Can you work these out from the model? Positions are in its coordinate system, mm. A direction names the side the tool comes from. Round coordinates to 2 decimals unless told otherwise and drop trailing zeros. Loops run counter-clockwise (first coordinate to the right, second up) from the corner with the lowest first, then second, coordinate; pieces in that order, holes last. Notation, with made-up numbers: M 56.25,62.5 L 104.25,62.5 A22 cw 104.25,87.5 Z; hole C 33.5,55.25 d1. An arc over 180 degrees is marked long. Return JSON: item names as keys, results as strings.
```python
from build123d import *

# Parameters (mm, degrees)
SKETCH_1_W             = 760
SKETCH_1_H             = 160
EXTRUDE_1_DEPTH        = 10
SKETCH_2_R             = 19
CUT_EXTRUDE_1_DEPTH    = 777.916983982
CUT_EXTRUDE_2_DEPTH    = 2
CUT_EXTRUDE_4_DEPTH    = 2.7
CUT_EXTRUDE_5_DEPTH    = 777.868071168
HOLE_WIZARD_M6_1_D     = 5
HOLE_WIZARD_M6_1_DEPTH = 15
HOLE_WIZARD_M6_1_TIP   = 1.502151548
FILLET_1_R             = 0.13
FILLET_2_R             = 0.5
FILLET_3_R             = 0.5
FILLET_4_R             = 0.13


with BuildPart() as part:
    # 스케치1 → 보스-돌출1 (new, symmetric)
    with BuildSketch(Plane(origin=(0, 0, 0), x_dir=(1, 0, 0), z_dir=(0, 1, 0))):
        with Locations((380, 80)):
            Rectangle(SKETCH_1_W, SKETCH_1_H)
    extrude(amount=EXTRUDE_1_DEPTH, both=True)

    # 스케치2 → 컷-돌출1 (cut, through all)
    with BuildSketch(Plane(origin=(0, 10, 0), x_dir=(1, 0, 0), z_dir=(0, 1, 0))):
        with Locations(Location((280, 80, 0), (0, 0, 270))):
            Circle(SKETCH_2_R)
        with Locations(Location((380, 80, 0), (0, 0, 270))):
            Circle(SKETCH_2_R)
    extrude(amount=-CUT_EXTRUDE_1_DEPTH, mode=Mode.SUBTRACT)

    # 스케치3 → 컷-돌출2 (cut)
    with BuildSketch(Plane(origin=(0, 10, 0), x_dir=(1, 0, 0), z_dir=(0, 1, 0))):
        with BuildLine():
            Line((520.5, 146), (679.5, 146))
            ThreePointArc((679.5, 146), (694.349242405, 139.849242405), (700.5, 125))
            Line((700.5, 125), (700.5, 66))
            ThreePointArc((700.5, 66), (694.349242405, 51.150757595), (679.5, 45))
            Line((679.5, 45), (520.5, 45))
            ThreePointArc((520.5, 45), (505.650757595, 51.150757595), (499.5, 66))
            Line((499.5, 66), (499.5, 125))
            ThreePointArc((499.5, 125), (505.650757595, 139.849242405), (520.5, 146))
        make_face()
    extrude(amount=-CUT_EXTRUDE_2_DEPTH, mode=Mode.SUBTRACT)

    # 스케치4 → 컷-돌출4 (cut)
    with BuildSketch(Plane(origin=(0, 8, 0), x_dir=(1, 0, 0), z_dir=(0, 1, 0))):
        with BuildLine():
            Line((532.5, 124.55), (667.5, 124.55))
            ThreePointArc((667.5, 124.55), (676.020636713, 121.020636713), (679.55, 112.5))
            Line((679.55, 112.5), (679.55, 77.5))
            ThreePointArc((679.55, 77.5), (676.020636713, 68.979363287), (667.5, 65.45))
            Line((667.5, 65.45), (532.5, 65.45))
            ThreePointArc((532.5, 65.45), (523.979363287, 68.979363287), (520.45, 77.5))
            Line((520.45, 77.5), (520.45, 112.5))
            ThreePointArc((520.45, 112.5), (523.979363287, 121.020636713), (532.5, 124.55))
        make_face()
        with BuildLine():
            Line((532.5, 120.45), (667.5, 120.45))
            ThreePointArc((667.5, 120.45), (673.12149891, 118.12149891), (675.45, 112.5))
            Line((675.45, 112.5), (675.45, 77.5))
            ThreePointArc((675.45, 77.5), (673.12149891, 71.87850109), (667.5, 69.55))
            Line((667.5, 69.55), (532.5, 69.55))
            ThreePointArc((532.5, 69.55), (526.87850109, 71.87850109), (524.55, 77.5))
            Line((524.55, 77.5), (524.55, 112.5))
            ThreePointArc((524.55, 112.5), (526.87850109, 118.12149891), (532.5, 120.45))
        make_face(mode=Mode.SUBTRACT)
    extrude(amount=-CUT_EXTRUDE_4_DEPTH, mode=Mode.SUBTRACT)

    # 스케치5 → 컷-돌출5 (cut, through all)
    with BuildSketch(Plane(origin=(0, 8, 0), x_dir=(1, 0, 0), z_dir=(0, 1, 0))):
        with BuildLine():
            Line((534.5, 116), (665.5, 116))
            ThreePointArc((665.5, 116), (669.035533906, 114.535533906), (670.5, 111))
            Line((670.5, 111), (670.5, 80))
            ThreePointArc((670.5, 80), (669.035533906, 76.464466094), (665.5, 75))
            Line((665.5, 75), (534.5, 75))
            ThreePointArc((534.5, 75), (530.964466094, 76.464466094), (529.5, 80))
            Line((529.5, 80), (529.5, 111))
            ThreePointArc((529.5, 111), (530.964466094, 114.535533906), (534.5, 116))
        make_face()
    extrude(amount=-CUT_EXTRUDE_5_DEPTH, mode=Mode.SUBTRACT)

    # M6 나사 구멍1
    with Locations(Plane(origin=(0, 8, 0), x_dir=(1, 0, 0), z_dir=(0, 1, 0))):
        with Locations((530, 135.5), (600, 135.5), (670, 135.5), (670, 54.5), (600, 54.5), (530, 54.5), (509.5, 95), (690.5, 95)):
            Hole(HOLE_WIZARD_M6_1_D / 2, depth=HOLE_WIZARD_M6_1_DEPTH)
            with Locations((0, 0, -(HOLE_WIZARD_M6_1_DEPTH + HOLE_WIZARD_M6_1_TIP / 2))):  # 118° drill point
                Cone(0, HOLE_WIZARD_M6_1_D / 2, HOLE_WIZARD_M6_1_TIP, mode=Mode.SUBTRACT)

    # 필렛1
    fillet_1_edges = [part.edges().sort_by_distance(p)[0] for p in [
        (523.979363287, 8, -121.020636713),
        (520.45, 8, -95),
        (523.979363287, 8, -68.979363287),
        (600, 8, -65.45),
        (676.020636713, 8, -68.979363287),
        (679.55, 8, -95),
        (676.020636713, 8, -121.020636713),
        (600, 8, -124.55),
    ]]
    fillet(fillet_1_edges, radius=FILLET_1_R)

    # 필렛2
    fillet_2_edges = [part.edges().sort_by_distance(p)[0] for p in [
        (523.979363287, 5.3, -121.020636713),
        (600, 5.3, -124.55),
        (676.020636713, 5.3, -121.020636713),
        (679.55, 5.3, -95),
        (676.020636713, 5.3, -68.979363287),
        (600, 5.3, -65.45),
        (523.979363287, 5.3, -68.979363287),
        (520.45, 5.3, -95),
    ]]
    fillet(fillet_2_edges, radius=FILLET_2_R)

    # 필렛3
    fillet_3_edges = [part.edges().sort_by_distance(p)[0] for p in [
        (675.45, 5.3, -95),
        (673.12149891, 5.3, -118.12149891),
        (600, 5.3, -120.45),
        (526.87850109, 5.3, -118.12149891),
        (524.55, 5.3, -95),
        (526.87850109, 5.3, -71.87850109),
        (600, 5.3, -69.55),
        (673.12149891, 5.3, -71.87850109),
    ]]
    fillet(fillet_3_edges, radius=FILLET_3_R)

    # 필렛4
    fillet_4_edges = [part.edges().sort_by_distance(p)[0] for p in [
        (673.12149891, 8, -118.12149891),
        (675.45, 8, -95),
        (673.12149891, 8, -71.87850109),
        (600, 8, -69.55),
        (526.87850109, 8, -71.87850109),
        (524.55, 8, -95),
        (526.87850109, 8, -118.12149891),
        (600, 8, -120.45),
    ]]
    fillet(fillet_4_edges, radius=FILLET_4_R)


solid = part.part
```
Q1. Suppose I cut it at C-C, the plane x = 368.5. Please give me the cut outline in (y, z).
Results:
{"outline": "M -10,-160 L 10,-160 L 10,-95.12 L -10,-95.12 Z; M -10,-64.88 L 10,-64.88 L 10,0 L -10,0 Z"}
Q2. Thinking about a two-plate mould opening in X: for faces 4 (the cylindrical face through (524.07, 6.85, -68.89)), 5 (the cylindrical face through (505.488, 9.014, -139.685)), 6 (the flat face through (0, 0, -79)), 7 (the flat face through (375, 0, -160)), which applies, pulls with the +X half, pulls with the -X half, needs draft (parallel to the pull), parting line crosses it, or undercut?
Results:
{"face 4": "undercut", "face 5": "undercut", "face 6": "pulls with the -X half", "face 7": "needs draft"}
Q3. Suppose I cut it at A-A, the plane y = -3.75. State how many separate pieces and enclosed holes the cut face has, plus the area to 3 significant figures.
Results:
{"separate pieces": "1", "enclosed holes": "11", "area": "113,000 mm2"}
Q4. If I drill on line 1 along X through (y, z) = (-1, -135.5); line 2 along X through (y, z) = (3.25, -55); line 3 along Z through (x, y) = (600, 1), over which ranges is the centre line in solid material (lowest first)?
Results:
{"line 1": "x = 0 to 527.5, 532.5 to 597.5, 602.5 to 667.5, 672.5 to 760", "line 2": "x = 0 to 527.55, 532.45 to 597.55, 602.45 to 667.55, 672.45 to 760", "line 3": "z = -160 to -138, -133 to -116, -75 to -57, -52 to 0"}
Q5. On a 3-axis mill with a long thin cutter (end or side, diameter ignored), from which of +Z, -Z, +X, -X, +Y, -Y can I reach the whole of each face in a straight line? I mean faces 1 (the flat face through (375, -10, -99)), 2 (the flat face through (670.5, -1, -96)), 3 (the cylindrical face through (676.11, 6.85, -69.07)). Say none if no direction works.
Results:
{"face 1": "+Z, -Z, +X, -X, -Y", "face 2": "+Y, -Y", "face 3": "+Y"}
Q6. I'm going to push flat-ended pins straight in: pin 1 Ø6 at (x, z) = (530, -135.5) entering from +Y; pin 2 Ø3 at (x, z) = (670, -135.5) entering from +Y. Where does each tip first touch, or does it pass through?
Results:
{"pin 1": "stops at y = 8", "pin 2": "stops at y = -7.6"}
Q7. Suppose I cut it at B-B, the plane x = 280. Please give me the cut outline in (y, z), plus the area to 3 significant figures.
Results:
{"outline": "M -10,-160 L 10,-160 L 10,-99 L -10,-99 Z; M -10,-61 L 10,-61 L 10,0 L -10,0 Z", "area": "2,440 mm2"}
